from build123d import *

# Parameters (mm, degrees)
F0_W     = 88.9
F0_H     = 127
F0_W_2   = 82.296
F0_H_2   = 53.654046
F0_H_3   = 63.439954
F1_DEPTH = 20.32
F2_DEPTH = 3.302
F3_W     = 1.27
F3_H     = 7.62
F3_W_2   = 7.62
F3_H_2   = 1.27
F4_DEPTH = 7.62
F5_R     = 1.143
F6_DEPTH = 1.271
F7_R     = 1.143
F8_DEPTH = 1.271


with BuildPart() as f1:
    # F0 (on Top) → F1 (new body)
    with BuildSketch(Plane.XY):
        with Locations((-17.722778, -0.396604)):
            Rectangle(F0_W, F0_H)
        with Locations((-17.722778, -33.767581)):
            Rectangle(F0_W_2, F0_H_2, mode=Mode.SUBTRACT)
        with Locations((-17.722778, 28.081419)):
            Rectangle(F0_W_2, F0_H_3, mode=Mode.SUBTRACT)
    extrude(amount=F1_DEPTH)

    # F0 (on Top) → F2 (join)
    with BuildSketch(Plane.XY):
        with Locations((-17.722778, -0.396604)):
            Rectangle(F0_W, F0_H)
        with Locations((-17.722778, -33.767581)):
            Rectangle(F0_W_2, F0_H_2, mode=Mode.SUBTRACT)
        with Locations((-17.722778, 28.081419)):
            Rectangle(F0_W_2, F0_H_3, mode=Mode.SUBTRACT)
        with Locations((-17.722778, 28.081419)):
            Rectangle(F0_W_2, F0_H_3)
        with Locations((-17.722778, -33.767581)):
            Rectangle(F0_W_2, F0_H_2)
    extrude(amount=-F2_DEPTH)

    # F3 (on face) → F4 (join)
    with BuildSketch(Plane.XY.offset(20.32)):
        with Locations((26.092222, 33.893396)):
            Rectangle(F3_W, F3_H)
        with Locations((-15.182778, -63.261604)):
            Rectangle(F3_W_2, F3_H_2)
    extrude(amount=F4_DEPTH)

    # F5 (on face) → F6 (cut, through all)
    with BuildSketch(Plane(origin=(0, -62.626604, 0), x_dir=(-1, 0, 0), z_dir=(0, 1, 0))):
        with Locations((15.182778, 24.13)):
            Circle(F5_R)
    extrude(amount=-F6_DEPTH, mode=Mode.SUBTRACT)

    # F7 (on face) → F8 (cut, through all)
    with BuildSketch(Plane(origin=(25.457222, 0, 0), x_dir=(0, -1, 0), z_dir=(-1, 0, 0))):
        with Locations((-33.893396, 24.13)):
            Circle(F7_R)
    extrude(amount=-F8_DEPTH, mode=Mode.SUBTRACT)


solid = f1.part
The model under review builds one solid part; all positions refer to its coordinate system, in mm. A direction names the side the tool comes from. Give positions to 0.01 mm unless a question says otherwise; leave off trailing zeros. Order: outer loops, then holes, each group sorted by start corner. A loop starts at its lowest first (then second) coordinate and runs counter-clockwise, first axis right, second up. Notation, with made-up numbers: (-29, -21.5) -> (25, -21.5) arc R25 ccw to (25, 11.5) -> close; hole circle Ø4 at (59, 25.5). An arc over 180 degrees is marked (long way). Write item = value, one per line. Start each with the question number.
(1) For L1, parallel to Y at x = -51.5, z = 3.5; L2, parallel to X at y = -55, z = 8; L3, parallel to X at y = -63, z = 24, list the stretches that pass through material, from the lowest coordinate up. Write a range as from..to.
(2) For pin 1 Ø1 at (y, z) = (-63, 22.5) entering from -X; pin 2 Ø1.4 at (x, z) = (26, 24.5) entering from +Y; pin 3 Ø0.6 at (x, z) = (26, 23) entering from -Y; pin 4 Ø1.4 at (y, z) = (33.89, 24.13) entering from +X, all flat-tipped, find the tip position at first contact; note any pin that passes through.
(3) Take a section at C-C (x = 14.5). Write out the cut boundary in (y, z).
(4) Tool access review of faces 1 (the flat face through (26.727, -1, 9)), 2 (the flat face through (-16, -62.627, 23)), 3 (the flat face through (-18, 63.103, 9)), 4 (the flat face through (-18, -60.595, 10)), 5 (the flat face through (25.457, 33, 23)): name each direction out of +Z, -Z, +X, -X, +Y, -Y from which nothing blocks a thin tool from reaching the whole face with its end or side.
(5) Draft analysis for pull direction X (two halves, no side actions). For faces 6 (the flat face through (-18, 0, -3.302)), 7 (the flat face through (-62.173, -1, 9)), 8 (the flat face through (-18, -6.941, 10)), state which applies: +X half, -X half, draft (parallel to the pull), parting line (faces both ways), or undercut.
(6) Take a section at B-B (y = 6). Write out the cut boundary in (x, z), plus the area to 3 significant figures.
(7) Take a section at A-A (z = 5.5). Write out the cut boundary in (x, y).
Returned:
q1.L1 = -63.9..-60.59, -6.94..-3.64, 59.8..63.1
q1.L2 = -62.17..-58.87, 23.43..26.73
q1.L3 = -18.99..-16.32, -14.05..-11.37
q2.pin_1 = -18.99
q2.pin_2 = 37.7
q2.pin_3 = 30.08
q2.pin_4 = through
q3.outline = (-63.9, -3.3) -> (63.1, -3.3) -> (63.1, 20.32) -> (59.8, 20.32) -> (59.8, 0) -> (-3.64, 0) -> (-3.64, 20.32) -> (-6.94, 20.32) -> (-6.94, 0) -> (-60.59, 0) -> (-60.59, 20.32) -> (-63.9, 20.32) -> close
q4.face_1 = +Z, -Z, +X, +Y, -Y
q4.face_2 = +Z, +X, -X, +Y
q4.face_3 = +Z, -Z, +X, -X, +Y
q4.face_4 = +Z
q4.face_5 = +Z, -X, +Y, -Y
q5.face_6 = draft
q5.face_7 = -X half
q5.face_8 = undercut
q6.outline = (-62.17, -3.3) -> (26.73, -3.3) -> (26.73, 20.32) -> (23.43, 20.32) -> (23.43, 0) -> (-58.87, 0) -> (-58.87, 20.32) -> (-62.17, 20.32) -> close
q6.area = 428 mm²
q7.outline = (-62.17, -63.9) -> (26.73, -63.9) -> (26.73, 63.1) -> (-62.17, 63.1) -> close; hole (-58.87, -60.59) -> (23.43, -60.59) -> (23.43, -6.94) -> (-58.87, -6.94) -> close; hole (-58.87, -3.64) -> (23.43, -3.64) -> (23.43, 59.8) -> (-58.87, 59.8) -> close
